Verification items for this drawing (mm, ordinates from the low corner). A direction names the side the tool comes from. Coordinates: 2 decimals unless noted, no trailing zeros. Order: outer loops, then holes, each group sorted by start corner. A loop starts at its lowest first (then second) coordinate and runs counter-clockwise, first axis right, second up. Notation, with made-up numbers: (-23, 10) -> (-3, 10) arc R18 cw to (-3, 26) -> close; hole circle Ø4 at (8.5, 60.25). An arc over 180 degrees is marked (long way). Write each question's results on one line, items separated by ' | '. Start each with the question number.
(1) Go/stop test with flat-tipped pins: pin 1 (1 mm diameter, centred on y = 2.5, z = 6.5, fed in from +X); pin 2 (2 mm diameter, centred on y = 10.5, z = 9, fed in from -X); pin 3 (2 mm diameter, centred on y = 1.5, z = 7, fed in from -X). Record where each tip stops, or that it passes through.
(2) Set-up check for the marked faces 5 and 6: record each of +Z, -Z, +X, -X, +Y, -Y from which the full face is reachable in a straight line by a thin tool's end or side.
(3) Draft check along X on the marked faces 1, 2, 3 and 4. Enter one of: +X half, -X half, draft (parallel to the pull), parting line (faces both ways), or undercut.
(4) Cross-section at B-B on x = 7. Enter the section's corners in (y, z), and give its area (3 significant figures).
(5) Thickness scan on probe 1 along X at (y, z) = (2, 7.5); probe 2 along Y at (x, z) = (7.5, 7.5); probe 3 along X at (y, z) = (13, 10.25) (1 decimal). Record the ranges inside material, lowest first. Write a range as [from, to].
(6) Cross-section at A-A on y = 3.5. Enter the section's corners in (x, z).
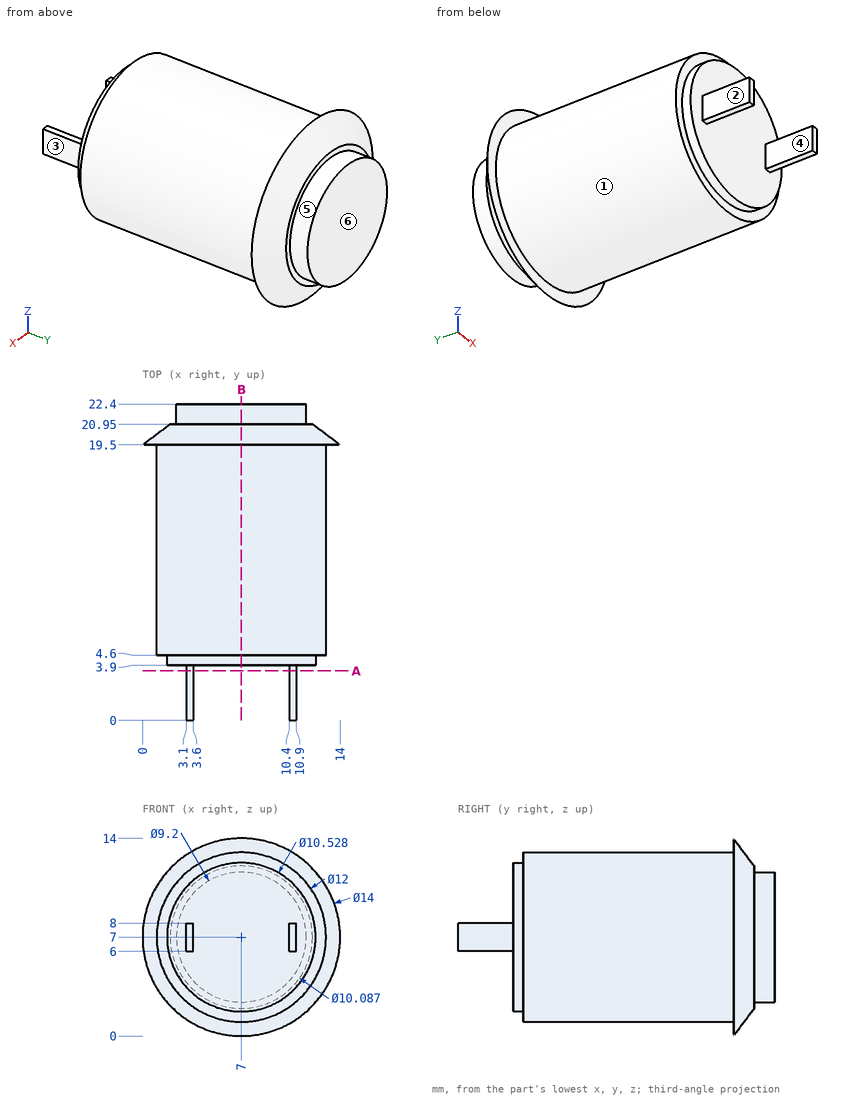
Results are:
1) pin 1: stops at x = 10.9 | pin 2: stops at x = 1.08 | pin 3: stops at x = 3.1
2) face 5: +Y | face 6: +Z, -Z, +X, -X, +Y
3) face 1: parting line | face 2: -X half | face 3: +X half | face 4: undercut
4) outline: (3.9, 1.74) -> (4.6, 1.74) -> (4.6, 1) -> (19.5, 1) -> (19.5, 0) -> (20.95, 1.96) -> (20.95, 2.4) -> (22.4, 2.4) -> (22.4, 11.6) -> (20.95, 11.6) -> (20.95, 12.04) -> (19.5, 14) -> (19.5, 13) -> (4.6, 13) -> (4.6, 12.26) -> (3.9, 12.26) -> close | area: 217 mm2
5) probe 1: x = [3.1, 3.6], [10.4, 10.9] | probe 2: y = [3.9, 22.4] | probe 3: x = [2, 12]
6) outline: (3.1, 6) -> (3.6, 6) -> (3.6, 8) -> (3.1, 8) -> close; (10.4, 6) -> (10.9, 6) -> (10.9, 8) -> (10.4, 8) -> close
